from build123d import *

# Parameters (mm, degrees)
ESQUISSE1_W             = 32.6
ESQUISSE1_H             = 34
BOSS_EXTRU_1_DEPTH      = 1
ESQUISSE2_W             = 5
ESQUISSE2_H             = 2.5
ESQUISSE2_W_2           = 15.2
ESQUISSE2_H_2           = 17.52
ESQUISSE2_W_3           = 3
ESQUISSE2_H_3           = 1
ESQUISSE2_H_4           = 2
BOSS_EXTRU_2_DEPTH      = 1
ESQUISSE3_W             = 15.2
ESQUISSE3_H             = 17.52
ESQUISSE3_W_2           = 5
ESQUISSE3_H_2           = 2.5
BOSS_EXTRU_3_DEPTH      = 1
ESQUISSE4_W             = 0.5
ESQUISSE4_H             = 2
ESQUISSE4_W_2           = 1.5
ESQUISSE4_H_2           = 0.5
ESQUISSE4_H_3           = 1.5
ESQUISSE4_W_3           = 3.5
ESQUISSE4_W_4           = 1
ESQUISSE4_H_4           = 1
ESQUISSE4_H_5           = 0.3
ESQUISSE4_W_5           = 0.553112931
ESQUISSE4_H_6           = 0.835313405
BOSS_EXTRU_4_DEPTH      = 1
ESQUISSE5_R             = 1
ESQUISSE5_R_2           = 0.75
BOSS_EXTRU_5_DEPTH      = 0.5
ESQUISSE6_R             = 1.9
ENL_V_MAT_EXTRU_1_DEPTH = 8.5
ESQUISSE7_W             = 18.1
ESQUISSE7_H             = 2.5
BOSS_EXTRU_6_DEPTH      = 2.5
BOSS_EXTRU_7_DEPTH      = 5
BOSS_EXTRU_7_DEPTH_BACK = 4
ESQUISSE8_R             = 0.25


with BuildPart() as part:
    # Esquisse1 → Boss.-Extru.1 (new body)
    with BuildSketch(Plane.XY):
        with Locations((-16.3, 17)):
            Rectangle(ESQUISSE1_W, ESQUISSE1_H)
    extrude(amount=BOSS_EXTRU_1_DEPTH)

    # Esquisse2 → Boss.-Extru.2 (add)
    with BuildSketch(Plane.XY.offset(1)):
        with Locations((-18.4, 28.05)):
            Rectangle(ESQUISSE2_W, ESQUISSE2_H)
        with Locations((-22.5, 16.04)):
            Rectangle(ESQUISSE2_W_2, ESQUISSE2_H_2)
        with Locations((-28.6, 6)):
            Rectangle(ESQUISSE2_W_3, ESQUISSE2_H_3)
        with Locations((-10.5, 9)):
            Rectangle(ESQUISSE2_W_3, ESQUISSE2_H_4)
        with Locations((-10.5, 6)):
            Rectangle(ESQUISSE2_W_3, ESQUISSE2_H_4)
    extrude(amount=BOSS_EXTRU_2_DEPTH)

    # Esquisse3 → Boss.-Extru.3 (add)
    with BuildSketch(Plane.XY.offset(2)):
        with Locations((-22.5, 16.04)):
            Rectangle(ESQUISSE3_W, ESQUISSE3_H)
        with Locations((-18.4, 28.05)):
            Rectangle(ESQUISSE3_W_2, ESQUISSE3_H_2)
    extrude(amount=BOSS_EXTRU_3_DEPTH)

    # Esquisse4 → Boss.-Extru.4 (add)
    with BuildSketch(Plane.XY.offset(1)):
        with Locations((-9.25, 13.5)):
            Rectangle(ESQUISSE4_W, ESQUISSE4_H)
        with Locations((-10.75, 13.5)):
            Rectangle(ESQUISSE4_W, ESQUISSE4_H)
        with Locations((-9.75, 17.75)):
            Rectangle(ESQUISSE4_W_2, ESQUISSE4_H_2)
        with Locations((-10.25, 24.816299889)):
            Rectangle(ESQUISSE4_W, ESQUISSE4_H_3)
        with Locations((-11.75, 24.816299889)):
            Rectangle(ESQUISSE4_W, ESQUISSE4_H_3)
        with Locations((-13.17709205, 30.55)):
            Rectangle(ESQUISSE4_W_3, ESQUISSE4_H_3)
        with Locations((-23.65, 28.699378422)):
            Rectangle(ESQUISSE4_W, ESQUISSE4_H_3)
        with Locations((-15.5, 5.633321931)):
            Rectangle(ESQUISSE4_W_4, ESQUISSE4_H_2)
        with Locations((-15.75, 4.133321931)):
            Rectangle(ESQUISSE4_W_2, ESQUISSE4_H_2)
        with Locations((-19, 3.221962501)):
            Rectangle(ESQUISSE4_W_4, ESQUISSE4_H)
        with Locations((-18.75, 5.918492514)):
            Rectangle(ESQUISSE4_W, ESQUISSE4_H_4)
        with Locations((-17.030226104, 3.13997626)):
            Rectangle(ESQUISSE4_W_2, ESQUISSE4_H_2)
        with Locations((-20.280226104, 3.13997626)):
            Rectangle(ESQUISSE4_W_4, ESQUISSE4_H_2)
        with Locations((-21.75, 4.471962501)):
            Rectangle(ESQUISSE4_W_2, ESQUISSE4_H_2)
        with Locations((-24, 4.53997626)):
            Rectangle(ESQUISSE4_W_4, ESQUISSE4_H_5)
        with Locations((-21.276556466, 6.400550167)):
            Rectangle(ESQUISSE4_W_5, ESQUISSE4_H_6)
    extrude(amount=BOSS_EXTRU_4_DEPTH)

    # Esquisse5 → Boss.-Extru.5 (add)
    with BuildSketch(Plane.XY.offset(1)):
        with Locations((-9, 21)):
            Circle(ESQUISSE5_R)
        with Locations((-9, 21)):
            Circle(ESQUISSE5_R_2, mode=Mode.SUBTRACT)
    extrude(amount=BOSS_EXTRU_5_DEPTH)

    # Esquisse6 → Enlèv. mat.-Extru.1 (cut)
    with BuildSketch(Plane.XY.offset(1)):
        with Locations((-30.6, 32)):
            Circle(ESQUISSE6_R)
        with Locations((-7, 32)):
            Circle(ESQUISSE6_R)
        with Locations((-7, 2.2)):
            Circle(ESQUISSE6_R)
    extrude(amount=-ENL_V_MAT_EXTRU_1_DEPTH, mode=Mode.SUBTRACT)

    # Esquisse7 → Boss.-Extru.6 (add)
    with BuildSketch(Plane(origin=(0, 0, 0), x_dir=(-1, 0, 0), z_dir=(0, 0, -1))):
        with Locations((21.05, 1.25)):
            Rectangle(ESQUISSE7_W, ESQUISSE7_H)
    extrude(amount=BOSS_EXTRU_6_DEPTH)

    # Esquisse8 → Boss.-Extru.7 (add, two sides: drawn at the far end of the back side and taken through both)
    with BuildSketch(Plane(origin=(0, 0, -2.5), x_dir=(-1, 0, 0), z_dir=(0, 0, -1)).offset(-BOSS_EXTRU_7_DEPTH_BACK)):
        with Locations((13.55, 1.25)):
            Circle(ESQUISSE8_R)
        with Locations((16.05, 1.25)):
            Circle(ESQUISSE8_R)
        with Locations((18.55, 1.25)):
            Circle(ESQUISSE8_R)
        with Locations((21.05, 1.25)):
            Circle(ESQUISSE8_R)
        with Locations((23.55, 1.25)):
            Circle(ESQUISSE8_R)
        with Locations((26.05, 1.25)):
            Circle(ESQUISSE8_R)
        with Locations((28.55, 1.25)):
            Circle(ESQUISSE8_R)
    extrude(amount=BOSS_EXTRU_7_DEPTH + BOSS_EXTRU_7_DEPTH_BACK)


solid = part.part
Geometry check sheet. Reference: the model listing, model coordinates, mm. A direction names the side the tool comes from. Give positions to 0.01 mm unless a question says otherwise; leave off trailing zeros. Loops run counter-clockwise (first coordinate to the right, second up) from the corner with the lowest first, then second, coordinate; pieces in that order, holes last. Notation, with made-up numbers: (20.5, 41) -> (42.5, 41) arc R11 cw to (42.5, 50) -> close; hole circle Ø10 at (22, 62.5). An arc over 180 degrees is marked (long way). Answer in a Markdown table with one row per item. Add a question column.
1) Cross-section at A-A on x = -30.6. Record the boundary of the cut face in (y, z), and give its area (3 significant figures).
2) Set-up check for faces 5 (the face through (-21.8, 4.222, 1.5)), 6 (the face through (-13.2, 29.8, 1.5)), 7 (the face through (-12, 1, -1)), 8 (the face through (-9, 13.5, 1.5)): record each of +Z, -Z, +X, -X, +Y, -Y from which the full face is reachable in a straight line by a thin tool's end or side.
3) Gauge pin test, flat ends, axial feed: P1, Ø1.5, axis at x = -16, z = -5, coming from the -Y side; P2, Ø0.6, axis at x = -19, z = 1.5, coming from the +Y side; P3, Ø0.5, axis at y = 13.5, z = 1.5, coming from the +X side. Record the tip position at first contact, or that the pin passes through.
4) Draft check along Y on faces 1 (the face through (-17, 17, 0)), 2 (the face through (-23, 7.28, 2)), 3 (the face through (-21.553, 6.4, 1.5)), 4 (the face through (-20, 0, 0)). Enter one of: pulls with the +Y half, pulls with the -Y half, needs draft (parallel to the pull), parting line crosses it, or undercut.
5) Cross-section at B-B on z = -5.75. Record the boundary of the cut face in (x, y).
6) Material ranges on probe 1 along Z at (x, y) = (-13, 18); probe 2 along Y at (x, z) = (-23.5, -2.25); probe 3 along Z at (x, y) = (-19, 27.5), recorded low to high. Write a range as from..to.
7) Cross-section at C-C on y = 32. Record the boundary of the cut face in (x, z), and give its area (3 significant figures).
8) Cross-section at D-D on x = -7. Record the boundary of the cut face in (y, z).
Outcome:
| question | item | result |
|---|---|---|
| 1 | outline | (0, 0) -> (30.1, 0) -> (30.1, 1) -> (0, 1) -> close; (33.9, 0) -> (34, 0) -> (34, 1) -> (33.9, 1) -> close |
| 1 | area | 30.2 mm^2 |
| 2 | face 5 | +Z, -X |
| 2 | face 6 | +Z, +X, -X |
| 2 | face 7 | -Z, +X, +Y, -Y |
| 2 | face 8 | +Z, +X, -Y |
| 3 | P1 | stops at y = 1 |
| 3 | P2 | stops at y = 29.3 |
| 3 | P3 | stops at x = -9 |
| 4 | face 1 | needs draft |
| 4 | face 2 | undercut |
| 4 | face 3 | undercut |
| 4 | face 4 | pulls with the -Y half |
| 5 | outline | circle Ø0.5 at (-28.55, 1.25); circle Ø0.5 at (-26.05, 1.25); circle Ø0.5 at (-23.55, 1.25); circle Ø0.5 at (-21.05, 1.25); circle Ø0.5 at (-18.55, 1.25); circle Ø0.5 at (-16.05, 1.25); circle Ø0.5 at (-13.55, 1.25) |
| 6 | probe 1 | z = 0..1 |
| 6 | probe 2 | y = 0..2.5 |
| 6 | probe 3 | z = 0..3 |
| 7 | outline | (-32.6, 0) -> (-32.5, 0) -> (-32.5, 1) -> (-32.6, 1) -> close; (-28.7, 0) -> (-8.9, 0) -> (-8.9, 1) -> (-28.7, 1) -> close; (-5.1, 0) -> (0, 0) -> (0, 1) -> (-5.1, 1) -> close |
| 7 | area | 25.0 mm^2 |
| 8 | outline | (0, 0) -> (0.3, 0) -> (0.3, 1) -> (0, 1) -> close; (4.1, 0) -> (30.1, 0) -> (30.1, 1) -> (4.1, 1) -> close; (33.9, 0) -> (34, 0) -> (34, 1) -> (33.9, 1) -> close |
